Read the model definition and answer for the solid it produces. Units are mm, in the model's axes. A direction names the side the tool comes from. Give positions to 0.01 mm unless a question says otherwise; leave off trailing zeros. Order: outer loops, then holes, each group sorted by start corner. A loop starts at its lowest first (then second) coordinate and runs counter-clockwise, first axis right, second up. Notation, with made-up numbers: (12, 16) - (70, 16) arc R28 cw to (70, 36) - close; hole circle Ø10 at (84.5, 73). An arc over 180 degrees is marked (long way). Return JSON: item names as keys, results as strings.
```python
from build123d import *

# Parameters (mm, degrees)
F0_R     = 15
F0_R_2   = 7.087313
F1_DEPTH = 25
F2_R     = 35


with BuildPart() as f1:
    # F0 (on Front) → F1 (new body)
    with BuildSketch(Plane.XZ):
        with BuildLine():
            add(Edge.make_bspline(
                [(0, 60.859382), (0, 26.312792), (0, 27.5), (-31.836466, 27.5)],
                knots=[0, 0, 0, 0, 46.113002, 46.113002, 46.113002, 46.113002], degree=3))
            Line((-31.836466, 27.5), (-153.096049, 27.5))
            ThreePointArc((-153.096049, 27.5), (-180.596049, 0), (-153.096049, -27.5))
            Line((-153.096049, -27.5), (-67.897924, -27.5))
            add(Edge.make_bspline(
                [(-67.897924, -27.5), (0, -27.5), (0, -27.5), (0, -89.587953)],
                knots=[0, 0, 0, 0, 92.005663, 92.005663, 92.005663, 92.005663], degree=3))
            Line((0, -89.587953), (0, -151.675906))
            ThreePointArc((0, -151.675906), (40, -191.675906), (80, -151.675906))
            Line((80, -151.675906), (80, -64.578305))
            add(Edge.make_bspline(
                [(111.659945, -24.140618), (80, -23.653816), (80, -23.971937), (80, -64.578305)],
                knots=[0, 0, 0, 0, 51.357167, 51.357167, 51.357167, 51.357167], degree=3))
            Line((111.659945, -24.140618), (111.659945, 60.859382))
            Line((111.659945, 60.859382), (0, 60.859382))
        make_face()
        with Locations((40, -151.675906)):
            Circle(F0_R, mode=Mode.SUBTRACT)
        with Locations((-125.648696, -13.373151)):
            Circle(F0_R_2, mode=Mode.SUBTRACT)
        with Locations((-59.283819, -13.373151)):
            Circle(F0_R_2, mode=Mode.SUBTRACT)
        with Locations((-125.648696, 13.373151)):
            Circle(F0_R_2, mode=Mode.SUBTRACT)
        with Locations((-59.283819, 13.373151)):
            Circle(F0_R_2, mode=Mode.SUBTRACT)
    extrude(amount=F1_DEPTH)

    # F2
    f2_edges = [f1.edges().sort_by_distance(p)[0] for p in [
        (111.659945, -12.5, 60.859382),
    ]]
    fillet(f2_edges, radius=F2_R)


solid = f1.part
```
Q1. Consider L1, parallel to Z at x = -126, y = -22.5; L2, parallel to Z at x = -63.5, y = -9.5; L3, parallel to X at y = -15.5, z = -10. Determine where each line is inside the solid, lowest interval first.
Values:
{"L1": "z = -27.5 to -20.45, -6.29 to 6.29, 20.45 to 27.5", "L2": "z = -27.5 to -19.07, -7.68 to 7.68, 19.07 to 27.5", "L3": "x = -178.71 to -131.88, -119.42 to -65.52, -53.05 to 111.66"}
Q2. Determine the mould class of faces 1 (the flat face through (39, -12, 60.859)), 2 (the flat face through (80, -12, -109)), 3 (the cylindrical face through (-66.364, -12.325, 13.685)) for opening direction Z: released by +Z, released by -Z, zero draft, split by the parting line, or undercut.
Values:
{"face 1": "released by +Z", "face 2": "zero draft", "face 3": "undercut"}
Q3. A cutting plane is placed at D-D (y = -6.25). Give the number of separate pieces and of enclosed holes in the cut face, and give its area (3 significant figures).
Values:
{"separate pieces": "1", "enclosed holes": "5", "area": "30,500 mm²"}
Q4. A cutting plane is placed at A-A (x = 40). Write down the section's boundary in (y, z).
Values:
{"outline": "(-25, -191.68) - (0, -191.68) - (0, -166.68) - (-25, -166.68) - close; (-25, -136.68) - (0, -136.68) - (0, 60.86) - (-25, 60.86) - close"}
Q5. Given pin 1 (7.5 mm diameter, centred on y = -9.5, z = -120, fed in from -X); pin 2 (12 mm diameter, centred on x = 3.5, y = -5, fed in from -Z); pin 3 (1 mm diameter, centred on y = -14.5, z = -126, fed in from +X), each flat-ended and moving along its own axis, determine where each tip first touches the part or whether it passes through.
Values:
{"pin 1": "stops at x = 0", "pin 2": "stops at z = -177.56", "pin 3": "stops at x = 80"}
Q6. A cutting plane is placed at C-C (z = -108). Write down the section's boundary in (x, y).
Values:
{"outline": "(0, -25) - (80, -25) - (80, 0) - (0, 0) - close"}
Q7. A cutting plane is placed at B-B (x = -123.5). Write down the section's boundary in (y, z).
Values:
{"outline": "(-25, -27.5) - (0, -27.5) - (0, -20.13) - (-25, -20.13) - close; (-25, -6.62) - (0, -6.62) - (0, 6.62) - (-25, 6.62) - close; (-25, 20.13) - (0, 20.13) - (0, 27.5) - (-25, 27.5) - close"}
Q8. For faces 4 (the flat face through (0, -12, -120)), 5 (the flat face through (-92, -12, 27.5)), 6 (the flat face through (-4, -25, -36)), determine the directions among +Z, -Z, +X, -X, +Y, -Y from which every point of the face is accessible in a straight line to the end or side of a thin tool.
Values:
{"face 4": "-Z, -X, +Y, -Y", "face 5": "+Z, -X, +Y, -Y", "face 6": "+Z, -Z, +X, -X, -Y"}
